Verification items for this drawing (mm, ordinates from the low corner). Round coordinates to 2 decimals unless told otherwise and drop trailing zeros. Order: outer loops, then holes, each group sorted by start corner. A loop starts at its lowest first (then second) coordinate and runs counter-clockwise, first axis right, second up. Notation, with made-up numbers: (81.5, 7) -> (129.5, 7) arc R25 cw to (129.5, 24) -> close; hole circle Ø9 at (-35, 22). An arc over 180 degrees is marked (long way). Return JSON: item names as keys, results as strings. Group by question number.
Item 1: Sectioned sample at C-C on z = 1.5. Record the cut outline in (x, y), plus the area to 3 significant figures.
Item 2: Draft check along Y on the marked faces 1, 2 and 3. Enter one of: pulls with the +Y half, pulls with the -Y half, needs draft (parallel to the pull), parting line crosses it, or undercut.
Item 3: Sectioned sample at B-B on y = 2.5. Record the cut outline in (x, z).
Item 4: Sectioned sample at D-D on y = 19.25. Record the cut outline in (x, z), plus the area to 3 significant figures.
Item 5: Scan lines: probe 1 along Y at (x, z) = (10.25, 3.3); probe 2 along X at (y, z) = (7.25, 3.9); probe 3 along X at (y, z) = (8.25, 4.65). Record each from-to range of solid material in increasing order. Write a range as from..to.
Item 6: Sectioned sample at A-A on x = 10.25. Record the cut outline in (y, z).
Item 7: Depth check by flat-ended pin: pin 1 Ø3 at (y, z) = (8, 3) entering from +X; pin 2 Ø2 at (y, z) = (15, 1) entering from -X. Enter the tip coordinate at first touch or a pass-through.
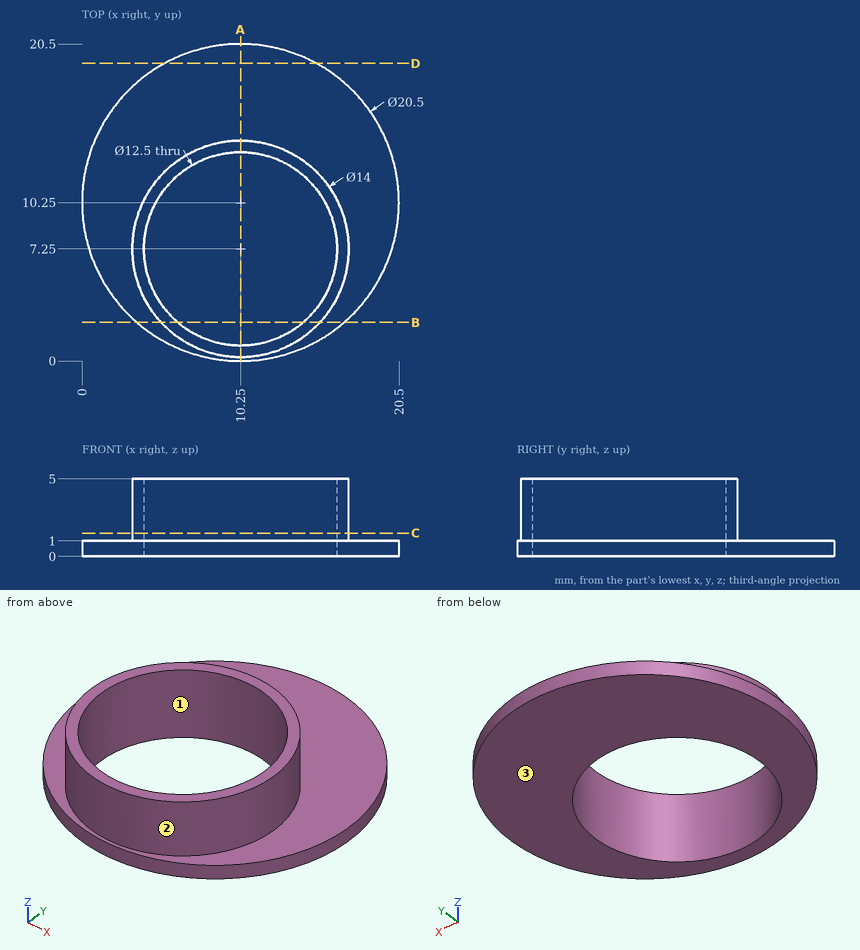
Recorded:
{
 "1": {"outline": "circle Ø14 at (10.25, 7.25); hole circle Ø12.5 at (10.25, 7.25)", "area": "31.2 mm²"},
 "2": {"face 1": "undercut", "face 2": "parting line crosses it", "face 3": "needs draft"},
 "3": {"outline": "(3.54, 0) -> (6.19, 0) -> (6.19, 5) -> (5.11, 5) -> (5.11, 1) -> (3.54, 1) -> close; (14.31, 0) -> (16.96, 0) -> (16.96, 1) -> (15.39, 1) -> (15.39, 5) -> (14.31, 5) -> close"},
 "4": {"outline": "(5.34, 0) -> (15.16, 0) -> (15.16, 1) -> (5.34, 1) -> close", "area": "9.81 mm²"},
 "5": {"probe 1": "0.25..1, 13.5..14.25", "probe 2": "3.25..4, 16.5..17.25", "probe 3": "3.32..4.08, 16.42..17.18"},
 "6": {"outline": "(0, 0) -> (1, 0) -> (1, 5) -> (0.25, 5) -> (0.25, 1) -> (0, 1) -> close; (13.5, 0) -> (20.5, 0) -> (20.5, 1) -> (14.25, 1) -> (14.25, 5) -> (13.5, 5) -> close"},
 "7": {"pin 1": "x = 17.25", "pin 2": "x = 0.71"}
}
